The model under review builds one solid part; all positions refer to its coordinate system, in mm. A direction names the side the tool comes from. Give positions to 0.01 mm unless a question says otherwise; leave off trailing zeros. Loops run counter-clockwise (first coordinate to the right, second up) from the corner with the lowest first, then second, coordinate; pieces in that order, holes last. Notation, with made-up numbers: M 41,66.25 L 66,66.25 A35 ccw 66,100.25 Z; hole C -9,82.5 d7. An arc over 180 degrees is marked long. Put each result on its own line as item: value. Start each with the question number.
```python
from build123d import *

# Parameters (mm, degrees)
SKETCH2_W                = 126
SKETCH2_H                = 215
BOSS_EXTRUDE1_DEPTH      = 86
BOSS_EXTRUDE2_DEPTH      = 10.5
BOSS_EXTRUDE2_DEPTH_BACK = 136.5
SKETCH3_W                = 5.3
SKETCH3_H                = 215
SKETCH5_R                = 2.8
CUT_EXTRUDE1_DEPTH       = 10.5
SKETCH6_R                = 2.8
CUT_EXTRUDE2_DEPTH       = 10.5
SKETCH7_R                = 2.8
CUT_EXTRUDE3_DEPTH       = 10.5
LPATTERN1_COUNT          = 2
LPATTERN1_PITCH          = 136.5
SKETCH8_W                = 126
SKETCH8_H                = 80.7
BOSS_EXTRUDE3_DEPTH      = 15


with BuildPart() as part:
    # Sketch2 → Boss-Extrude1 (new body)
    with BuildSketch(Plane.XY):
        with Locations((63, 107.5)):
            Rectangle(SKETCH2_W, SKETCH2_H)
    extrude(amount=BOSS_EXTRUDE1_DEPTH)

    # Sketch3 → Boss-Extrude2 (add, two sides: drawn at the far end of the back side and taken through both)
    with BuildSketch(Plane(origin=(126, 0, 0), x_dir=(0, 0, -1), z_dir=(1, 0, 0)).offset(-BOSS_EXTRUDE2_DEPTH_BACK)):
        with Locations((-2.65, 107.5)):
            Rectangle(SKETCH3_W, SKETCH3_H)
    extrude(amount=BOSS_EXTRUDE2_DEPTH + BOSS_EXTRUDE2_DEPTH_BACK)

    # Sketch5 → Cut-Extrude1 (cut)
    with BuildSketch(Plane.XY.offset(5.3)):
        with Locations((131.25, 28)):
            Circle(SKETCH5_R)
    cut_extrude1 = extrude(amount=-CUT_EXTRUDE1_DEPTH, mode=Mode.SUBTRACT)

    # Sketch6 → Cut-Extrude2 (cut)
    with BuildSketch(Plane.XY.offset(5.3)):
        with Locations((131.25, 107.5)):
            Circle(SKETCH6_R)
    cut_extrude2 = extrude(amount=-CUT_EXTRUDE2_DEPTH, mode=Mode.SUBTRACT)

    # Sketch7 → Cut-Extrude3 (cut)
    with BuildSketch(Plane.XY.offset(5.3)):
        with Locations((131.25, 187)):
            Circle(SKETCH7_R)
    cut_extrude3 = extrude(amount=-CUT_EXTRUDE3_DEPTH, mode=Mode.SUBTRACT)

    # LPattern1: Cut-Extrude1, Cut-Extrude2, Cut-Extrude3 ×2
    with Locations(*[(-i * LPATTERN1_PITCH, 0, 0) for i in range(1, LPATTERN1_COUNT)]):
        add(cut_extrude1, mode=Mode.SUBTRACT)
        add(cut_extrude2, mode=Mode.SUBTRACT)
        add(cut_extrude3, mode=Mode.SUBTRACT)

    # Sketch8 → Boss-Extrude3 (add)
    with BuildSketch(Plane(origin=(0, 215, 0), x_dir=(1, 0, 0), z_dir=(0, 1, 0))):
        with Locations((63, -45.65)):
            Rectangle(SKETCH8_W, SKETCH8_H)
    extrude(amount=BOSS_EXTRUDE3_DEPTH)


solid = part.part
```
Item 1: Consider section B-B, the plane x = -5.25. Write out the cut boundary in (y, z), plus the area to 3 significant figures.
Item 2: Consider section C-C, the plane y = 158. Write out the cut boundary in (x, z).
Item 3: Consider section D-D, the plane z = 19. Write out the cut boundary in (x, y).
Item 4: Draft analysis for pull direction X (two halves, no side actions). For faces 4 (the flat face through (62, 222, 5.3)), 5 (the cylindrical face through (-7.314, 29.892, 2.687)), 6 (the flat face through (136.5, 109, 3)), state which applies: +X half, -X half, draft (parallel to the pull), parting line (faces both ways), or undercut.
Item 5: To check wall thickness, follow L1, parallel to Y at x = 131.25, z = 2.95; L2, parallel to X at y = 187, z = 2; L3, parallel to X at y = 59, z = 52.5. State the ranges of each line that lie inside material, in increasing order. Write a range as [from, to].
Item 6: Tool access review of faces 1 (the flat face through (62, 215, 3)), 2 (the flat face through (126, 113, 46)), 3 (the flat face through (-8, 106, 5.3)): name each direction out of +Z, -Z, +X, -X, +Y, -Y from which nothing blocks a thin tool from reaching the whole face with its end or side.
Item 7: Consider section A-A, the plane y = 107.5. Write out the cut boundary in (x, z), plus the area to 3 significant figures.
Item 8: Clearance check with flat-ended pins moving along their axes: pin 1 Ø5 at (x, y) = (-5.5, 69) entering from +Z; pin 2 Ø24 at (y, z) = (151.5, 43.5) entering from -X; pin 3 Ø1 at (y, z) = (110, 75) entering from +X. State where each tip first meets the part, or that it passes through.
Report:
1. outline: M 0,0 L 25.2,0 L 25.2,5.3 L 0,5.3 Z; M 30.8,0 L 104.7,0 L 104.7,5.3 L 30.8,5.3 Z; M 110.3,0 L 184.2,0 L 184.2,5.3 L 110.3,5.3 Z; M 189.8,0 L 215,0 L 215,5.3 L 189.8,5.3 Z
1. area: 1,050 mm²
2. outline: M -10.5,0 L 136.5,0 L 136.5,5.3 L 126,5.3 L 126,86 L 0,86 L 0,5.3 L -10.5,5.3 Z
3. outline: M 0,0 L 126,0 L 126,230 L 0,230 Z
4. face 4: draft
4. face 5: undercut
4. face 6: +X half
5. L1: [0, 25.2], [30.8, 104.7], [110.3, 184.2], [189.8, 215]
5. L2: [-10.5, -8.05], [-2.45, 128.45], [134.05, 136.5]
5. L3: [0, 126]
6. face 1: -Z, +X, -X, +Y
6. face 2: +Z, +X, +Y, -Y
6. face 3: +Z, -X, +Y, -Y
7. outline: M -10.5,0 L -8.05,0 L -8.05,5.3 L -10.5,5.3 Z; M -2.45,0 L 128.45,0 L 128.45,5.3 L 126,5.3 L 126,86 L 0,86 L 0,5.3 L -2.45,5.3 Z; M 134.05,0 L 136.5,0 L 136.5,5.3 L 134.05,5.3 Z
7. area: 10,900 mm²
8. pin 1: z = 5.3
8. pin 2: x = 0
8. pin 3: x = 126
